Can you work these out from the model? Positions are in its coordinate system, mm. Coordinates: 2 decimals unless noted, no trailing zeros. Order: outer loops, then holes, each group sorted by start corner. A loop starts at its lowest first (then second) coordinate and runs counter-clockwise, first axis right, second up. Notation, with made-up numbers: M -28,-14 L 19,-14 A21 cw 19,7 Z; hole C 47,56 d8. An arc over 180 degrees is marked long. Answer as a JSON object with one key per item and string values.
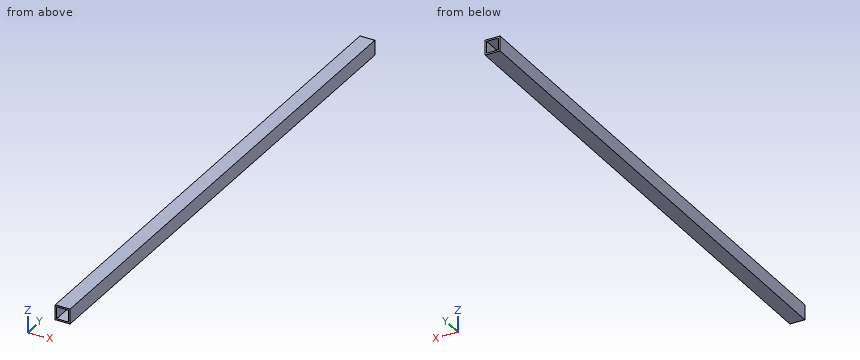
Autodesk Inventor part; units mm, degrees
ref_plane "YZ Plane" through (0, 0, 0) normal (1, 0, 0) x (0, 1, 0)
ref_plane "XZ Plane" through (0, 0, 0) normal (0, 1, 0) x (-1, 0, 0)
ref_plane "XY Plane" through (0, 0, 0) normal (0, 0, 1) x (1, 0, 0)
sketch "Sketch1" plane through (0, 0, 0) normal (0, 1, 0) x (-1, 0, 0)
  line L0 (15.875, 15.875) -> (-15.875, 15.875)
  line L1 (-15.875, 15.875) -> (-15.875, -15.875)
  line L2 (-15.875, -15.875) -> (15.875, -15.875)
  line L3 (15.875, -15.875) -> (15.875, 15.875)
  line L4 (15.875, 15.875) -> (-15.875, -15.875) construction
  line L5 (-15.875, 15.875) -> (15.875, -15.875) construction
  line L6 (12.7, 12.7) -> (-12.7, 12.7)
  line L7 (-12.7, 12.7) -> (-12.7, -12.7)
  line L8 (-12.7, -12.7) -> (12.7, -12.7)
  line L9 (12.7, -12.7) -> (12.7, 12.7)
  line L10 (12.7, 12.7) -> (-12.7, -12.7) construction
  line L11 (-12.7, 12.7) -> (12.7, -12.7) construction
  point P0 (0, 0)
  dimension "d0" = 31.75
  dimension "d1" = 3.175
extrude "Extrusion1" add sketch "Sketch1" along normal blind 1143
equation "\"d0\" = tubeSize"
equation "\"d1\" = tubeThickness"
equation "\"d2\" = tubeLength"
equation "\"tubeSize\" = 31.75"
equation "\"tubeThickness\" = 3.175"
equation "\"tubeLength\" = 1143"
properties part number "1_250_inchSquareTube" material "Aluminum 6061"
Item 1: I want a section at B-B, the plane x = -1.5. Write out the boundary of the cut face in (y, z) (3 decimals).
Answers follow:
{"outline": "M 0,-15.875 L 1143,-15.875 L 1143,-12.7 L 0,-12.7 Z; M 0,12.7 L 1143,12.7 L 1143,15.875 L 0,15.875 Z"}
Item 2: I want a section at A-A, the plane y = 427.5. Write out the boundary of the cut face in (x, z) (3 decimals), plus the area to 3 significant figures.
Answers follow:
{"outline": "M -15.875,-15.875 L 15.875,-15.875 L 15.875,15.875 L -15.875,15.875 Z; hole M -12.7,-12.7 L 12.7,-12.7 L 12.7,12.7 L -12.7,12.7 Z", "area": "363 mm^2"}
Item 3: Please list where this line runs through material, in increasing order: line 1 (Z direction, x = 6, y = 129) (3 decimals).
Answers follow:
{"line 1": "z = -15.875 to -12.7, 12.7 to 15.875"}
Item 4: I want a section at C-C, the plane z = -7. Write out the boundary of the cut face in (x, y) (3 decimals), plus the area to 3 significant figures.
Answers follow:
{"outline": "M -15.875,0 L -12.7,0 L -12.7,1143 L -15.875,1143 Z; M 12.7,0 L 15.875,0 L 15.875,1143 L 12.7,1143 Z", "area": "7,260 mm^2"}
